Autodesk Inventor part; units mm, degrees
ref_plane "YZ Plane" through (0, 0, 0) normal (1, 0, 0) x (0, 1, 0)
ref_plane "XZ Plane" through (0, 0, 0) normal (0, 1, 0) x (-1, 0, 0)
ref_plane "XY Plane" through (0, 0, 0) normal (0, 0, 1) x (1, 0, 0)
sketch "Sketch1" plane through (0, 0, 0) normal (0, 0, 1) x (1, 0, 0)
  circle A0 centre (-38.3507, 10.1677) radius 10.4
  line L0 (-51.23, -10.8726) -> (-51.1921, -10.9035)
  line L1 (-51.1921, -10.9035) -> (-36.539, -7.9419)
  line L2 (-36.539, -7.9419) -> (-21.5895, -7.9419)
  line L3 (-21.5895, -7.9419) -> (-13.5401, -14.5272)
  line L4 (-9.2136, -9.2389) -> (-13.5401, -14.5272)
  line L5 (-17.2631, -2.6536) -> (-9.2136, -9.2389)
  line L6 (-17.2631, -2.6536) -> (-17.2795, -2.6737)
  line L7 (-17.2795, -2.6737) -> (-20.2411, 11.9795)
  line L8 (-20.2411, 11.9795) -> (-20.2411, 26.9289)
  line L9 (-20.2411, 26.9289) -> (-13.6558, 34.9784)
  line L10 (-18.9241, 39.2883) -> (-13.6558, 34.9784)
  line L11 (-25.5094, 31.2389) -> (-18.9241, 39.2883)
  line L12 (-25.5094, 31.2389) -> (-40.1625, 28.2773)
  line L13 (-40.1625, 28.2773) -> (-55.3133, 28.2773)
  line L14 (-55.3133, 28.2773) -> (-55.2326, 28.3759)
  line L15 (-55.2326, 28.3759) -> (-63.282, 34.9612)
  line L16 (-67.592, 29.693) -> (-63.282, 34.9612)
  line L17 (-59.5426, 23.1077) -> (-67.592, 29.693)
  line L18 (-59.5426, 23.1077) -> (-59.4618, 23.2064)
  line L19 (-59.4618, 23.2064) -> (-56.4603, 8.3559)
  line L20 (-56.4603, 8.3559) -> (-56.4603, -6.5936)
  line L21 (-56.4603, -6.5936) -> (-63.0456, -14.643)
  line L22 (-57.8153, -18.922) -> (-63.0456, -14.643)
  line L23 (-51.23, -10.8726) -> (-57.8153, -18.922)
  circle A1 centre (-38.3507, 10.1677) radius 10.4
  line L24 (-51.23, -10.8726) -> (-51.1921, -10.9035)
  line L25 (-51.1921, -10.9035) -> (-36.539, -7.9419)
  line L26 (-36.539, -7.9419) -> (-21.5895, -7.9419)
  line L27 (-21.5895, -7.9419) -> (-13.5401, -14.5272)
  line L28 (-9.2136, -9.2389) -> (-13.5401, -14.5272)
  line L29 (-17.2631, -2.6536) -> (-9.2136, -9.2389)
  line L30 (-17.2631, -2.6536) -> (-17.2795, -2.6737)
  line L31 (-17.2795, -2.6737) -> (-20.2411, 11.9795)
  line L32 (-20.2411, 11.9795) -> (-20.2411, 26.9289)
  line L33 (-20.2411, 26.9289) -> (-13.6558, 34.9784)
  line L34 (-18.9241, 39.2883) -> (-13.6558, 34.9784)
  line L35 (-25.5094, 31.2389) -> (-18.9241, 39.2883)
  line L36 (-25.5094, 31.2389) -> (-40.1625, 28.2773)
  line L37 (-40.1625, 28.2773) -> (-55.3133, 28.2773)
  line L38 (-55.3133, 28.2773) -> (-55.2326, 28.3759)
  line L39 (-55.2326, 28.3759) -> (-63.282, 34.9612)
  line L40 (-67.592, 29.693) -> (-63.282, 34.9612)
  line L41 (-59.5426, 23.1077) -> (-67.592, 29.693)
  line L42 (-59.5426, 23.1077) -> (-59.4618, 23.2064)
  line L43 (-59.4618, 23.2064) -> (-56.4603, 8.3559)
  line L44 (-56.4603, 8.3559) -> (-56.4603, -6.5936)
  line L45 (-56.4603, -6.5936) -> (-63.0456, -14.643)
  line L46 (-57.8153, -18.922) -> (-63.0456, -14.643)
  line L47 (-51.23, -10.8726) -> (-57.8153, -18.922)
  point P0 (0, 0)
extrude "Extrusion1" add sketch "Sketch1" along normal blind 70.935
sketch "Sketch2" plane through (-59.5426, 23.1077, 0) normal (-0.6332026, -0.7739861, 0) x (0.7739861, -0.6332026, 0)
  line L0 (47.2215, 0) -> (47.2215, 55.335)
  line L1 (49.0358, 0) -> (49.0358, 70.935)
  line L2 (49.0358, 55.335) -> (60.717, 55.335)
  line L3 (60.717, 55.335) -> (60.717, 0)
  line L4 (60.717, 0) -> (49.0358, 0)
extrude "Extrusion2" cut sketch "Sketch2" against normal blind 70.935
sketch "Sketch3" plane through (-13.6558, 34.9784, 70.935) normal (0.7739861, -0.6332026, 0) x (0, 0, -1)
  line L0 (70.935, -21.9707) -> (70.935, -10.4)
  line L1 (70.935, -10.4) -> (15.6, -10.4)
  line L2 (70.935, -10.4) -> (0, -10.4)
  line L3 (15.6, -10.4) -> (15.6, 1.2922)
  line L4 (15.6, 1.2922) -> (70.935, 1.2922)
  line L5 (70.935, 1.2922) -> (70.935, -10.4)
  point P0 (70.935, -18.4258)
extrude "Extrusion3" cut sketch "Sketch3" against normal blind 70.935
sketch "Sketch5" plane through (-63.282, 34.9612, 70.935) normal (0.6332026, 0.7739861, 0) x (0.7739861, -0.6332026, 0)
  line L0 (0, 70.935) -> (0, 0)
  line L1 (0, 70.935) -> (0, 15.6)
  line L2 (0, 15.6) -> (10.4, 15.6)
  line L3 (10.4, 70.935) -> (10.4, 0)
  line L4 (10.4, 15.6) -> (10.4, 70.935)
  line L5 (10.4, 70.935) -> (0, 70.935)
  point P0 (71.117, 70.935)
  point P1 (10.4, 15.6)
extrude "Extrusion4" cut sketch "Sketch5" against normal blind 70.935
sketch "Sketch6" plane through (-63.0456, -14.643, 0) normal (-0.7739861, 0.6332026, 0) x (0, 0, 1)
  line L0 (0, 0) -> (0, 10.4)
  line L1 (0, 0) -> (55.335, 0)
  line L2 (0, 0) -> (70.935, 0)
  line L3 (55.335, 0) -> (55.335, 10.4601)
  line L4 (55.335, 10.4601) -> (0, 10.4601)
  line L5 (0, 10.4601) -> (0, 0)
  point P0 (0, 51.2542)
extrude "Extrusion5" cut sketch "Sketch6" against normal blind 70.935
sketch "Sketch7" plane through (-13.6558, 34.9784, 70.935) normal (0.7739861, -0.6332026, 0) x (0, 0, -1)
  circle A0 centre (5.281, -5.0747) radius 1.841
  point P0 (70.935, -18.4258)
extrude "Extrusion6" cut sketch "Sketch7" against normal blind 70.935
sketch "Sketch8" plane through (-51.23, -10.8726, 70.935) normal (0.7739861, -0.6332026, 0) x (0, 0, -1)
  circle A0 centre (5.0992, -4.9107) radius 1.841
  point P0 (70.935, 40.8542)
extrude "Extrusion7" cut sketch "Sketch8" against normal blind 70.935
sketch "Sketch9" plane through (-13.5401, -14.5272, 55.335) normal (-0.6332026, -0.7739861, 0) x (0.7739861, -0.6332026, 0)
  circle A0 centre (-5.0967, 11.2282) radius 1.841
  circle A1 centre (-64.9486, 11.2282) radius 1.841
  point P0 (1.2811, -55.335)
extrude "Extrusion8" cut sketch "Sketch9" against normal blind 70.935
sketch "Sketch10" plane through (0, 0, 0) normal (0, 0, -1) x (-1, 0, 0)
  line L0 (22.3279, -5.5568) -> (19.104, -2.4278)
  line L1 (19.104, -2.4278) -> (23.2761, 11.2262)
  line L2 (23.2761, 11.2262) -> (23.2761, 26.1128)
  arc A0 (26.1681, 28.9573) -> (23.2761, 26.1128) centre (26.1211, 26.1128) ccw
  line L3 (26.1681, 28.9573) -> (40.1539, 26.1128)
  line L4 (40.1539, 26.1128) -> (53.066, 26.1128)
  line L5 (53.066, 26.1128) -> (56.4891, 22.7904)
  line L6 (50.9259, -7.8719) -> (54.7765, -5.1545)
  line L7 (54.7765, -5.1545) -> (54.7765, 8.6166)
  line L8 (54.7765, 8.6166) -> (56.4881, 23.4995)
  line L9 (51.7835, -7.2666) -> (36.3702, -5.5568)
  line L10 (36.3702, -5.5568) -> (22.3279, -5.5568)
  circle A1 centre (38.1545, 10.5282) radius 13.3756
  point P0 (0, 0)
  point P1 (56.4148, 22.8625)
extrude "Extrusion9" cut sketch "Sketch10" against normal blind 64
properties part number "Lifter compartment"
Geometry check sheet. Reference: the model listing, model coordinates, mm. A direction names the side the tool comes from. Give positions to 0.01 mm unless a question says otherwise; leave off trailing zeros. Write each loop counter-clockwise with the first axis right and the second up, starting at its lowest first coordinate (ties: lowest second). Pieces come first, ordered by that corner, then holes.
1) Go/stop test with flat-tipped pins: pin 1 Ø8 at (y, z) = (17.5, 31.5) entering from -X; pin 2 Ø16.5 at (x, z) = (-51.5, 20) entering from +Y; pin 3 Ø10.5 at (x, z) = (-48, 18.5) entering from -Y; pin 4 Ø8 at (x, y) = (-37.5, 15) entering from +Z. Record where each tip stops, or that it passes through.
Values follow:
pin 1: stops at x = -59.12
pin 2: stops at y = 28.28
pin 3: stops at y = -10.89
pin 4: passes through
2) Cross-section at B-B (z = 20.5). Record the boundary of the cut face in (x, y), plus the area to 3 significant figures.
Values follow:
outline: (-59.46, 23.21) - (-56.46, 8.36) - (-56.46, -6.59) - (-56.42, -6.55) - (-51.12, -10.89) - (-36.54, -7.94) - (-21.59, -7.94) - (-17.28, -2.67) - (-20.24, 11.98) - (-20.24, 26.93) - (-25.51, 31.24) - (-40.16, 28.28) - (-55.31, 28.28) - close; circle Ø26.75 at (-38.15, 10.53); hole (-56.41, 22.86) - (-54.78, 8.62) - (-54.78, -5.15) - (-51.78, -7.27) - (-36.37, -5.56) - (-22.33, -5.56) - (-19.1, -2.43) - (-23.28, 11.23) - (-23.28, 26.11) arc R2.85 ccw to (-26.17, 28.96) - (-40.15, 26.11) - (-53.07, 26.11) - close; hole circle Ø20.8 at (-38.35, 10.17)
area: 551 mm2
3) Cross-section at C-C (y = 6). Record the boundary of the cut face in (x, z) (1 decimal).
Values follow:
outline: (-56.5, 0) - (-54.8, 0) - (-54.8, 64) - (-50.7, 64) - (-50.7, 0) - (-47.9, 0) - (-47.9, 70.9) - (-56.5, 70.9) - close; (-28.8, 0) - (-25.6, 0) - (-25.6, 64) - (-21.7, 64) - (-21.7, 0) - (-19, 0) - (-19, 70.9) - (-28.8, 70.9) - close
4) Set-up check for faces 1 (the face through (-54.477, -14.841, 63.026)), 2 (the face through (-53.807, -8.687, 28.055)), 3 (the face through (-54.776, 2, 32)): record each of +Z, -Z, +X, -X, +Y, -Y from which the full face is reachable in a straight line by a thin tool's end or side.
Values follow:
face 1: +Z, -Z, -Y
face 2: -Z, -X, -Y
face 3: -Z
5) Cross-section at A-A (x = -34.5). Record the boundary of the cut face in (y, z) (3 decimals).
Values follow:
outline: (-7.942, 0) - (-5.557, 0) - (-5.557, 64) - (-2.338, 64) - (-2.338, 0) - (0.507, 0) - (0.507, 70.935) - (-7.942, 70.935) - close; (19.829, 0) - (23.395, 0) - (23.395, 64) - (27.263, 64) - (27.263, 0) - (29.422, 0) - (29.422, 70.935) - (19.829, 70.935) - close
6) Thickness scan on line 1 (X direction, y = 3.5, z = 54.5); line 2 (Y direction, x = -30, z = 47); line 3 (Y direction, x = -29, z = 63.5). Record the ranges inside material, lowest first.
Values follow:
line 1: x = -56.46 to -54.78, -49.53 to -46.33, -30.37 to -26.77, -20.92 to -18.53
line 2: y = -7.94 to -5.56, -0.07 to 3.97, 16.37 to 21.13, 28.18 to 30.33
line 3: y = -7.94 to -5.56, 0.78 to 5.62, 14.72 to 20.28, 28.38 to 30.53
7) Release check for a two-part mould opening along Y. For faces 4 (the face through (-11.35, -11.85, 63.03)), 5 (the face through (-32.73, 29.78, 34.97)), 6 (the face through (-59.707, -10.562, 63.026)) record: released by +Y, released by -Y, zero draft, split by the parting line, or undercut.
Values follow:
face 4: released by -Y
face 5: released by +Y
face 6: undercut
